```python
from build123d import *

# Parameters (mm, degrees)
ESQUISSE1_W        = 90
ESQUISSE1_H        = 250
BOSS_EXTRU_1_DEPTH = 5
ESQUISSE2_W        = 90
ESQUISSE2_H        = 250
ESQUISSE2_W_2      = 80
ESQUISSE2_H_2      = 240
BOSS_EXTRU_2_DEPTH = 75
BOSS_EXTRU_3_DEPTH = 5


with BuildPart() as part:
    # Esquisse1 → Boss.-Extru.1 (new body)
    with BuildSketch(Plane.XY):
        with Locations((-45, 125)):
            Rectangle(ESQUISSE1_W, ESQUISSE1_H)
    extrude(amount=BOSS_EXTRU_1_DEPTH)

    # Esquisse2 → Boss.-Extru.2 (add)
    with BuildSketch(Plane(origin=(0, 0, 0), x_dir=(-1, 0, 0), z_dir=(0, 0, -1))):
        with Locations((45, 125)):
            Rectangle(ESQUISSE2_W, ESQUISSE2_H)
        with Locations((45, 125)):
            Rectangle(ESQUISSE2_W_2, ESQUISSE2_H_2, mode=Mode.SUBTRACT)
    extrude(amount=BOSS_EXTRU_2_DEPTH)

    # Esquisse3 → Boss.-Extru.3 (add)
    with BuildSketch(Plane(origin=(0, 0, -75), x_dir=(-1, 0, 0), z_dir=(0, 0, -1))):
        Polygon((6.025463364, 250), (-96.347652867, 250), (-96.347652867, 0), (-31.347652867, 0), (45, 0), (45, 5), (5, 5), (5, 245), (45, 245), (45, 250), align=None)
    boss_extru_3 = extrude(amount=BOSS_EXTRU_3_DEPTH)

    # Symétrie1: Boss.-Extru.3 across plane
    add(boss_extru_3.mirror(Plane(origin=(-45, 245, -80), x_dir=(0, 0, 1), z_dir=(1, 0, 0))))


solid = part.part
```
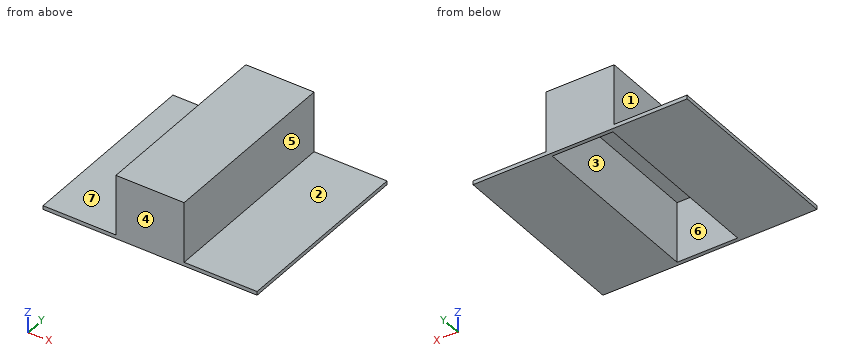
Source: CAD feature listing. Evaluate the final solid. Frame: model axes, mm. Face numbers are marked on the shaded views. A direction names the side the tool comes from. Give positions to 0.01 mm unless a question says otherwise; leave off trailing zeros. Order: outer loops, then holes, each group sorted by start corner. A loop starts at its lowest first (then second) coordinate and runs counter-clockwise, first axis right, second up. Notation, with made-up numbers: (50.5, -29.5) -> (105.5, -29.5) arc R12 ccw to (105.5, -7.5) -> close; hole circle Ø7 at (85, 76). An arc over 180 degrees is marked (long way). Use a Markdown table: item, result.
Q1. Section B-B (y = 50). Return the cut outline in (x, z).
A:
| item | result |
|---|---|
| outline | (-186.35, -80) -> (-85, -80) -> (-85, 0) -> (-5, 0) -> (-5, -80) -> (96.35, -80) -> (96.35, -75) -> (0, -75) -> (0, 5) -> (-90, 5) -> (-90, -75) -> (-186.35, -75) -> close |
Q2. Material intervals for line 1 (X direction, y = 39, z = -30.5); line 2 (Y direction, x = -8, z = -16.5); line 3 (Z direction, x = -44, y = 193.5), sorted ascending. Write a range as [from, to].
A:
| item | result |
|---|---|
| line 1 | [-90, -85], [-5, 0] |
| line 2 | [0, 5], [245, 250] |
| line 3 | [0, 5] |
Q3. Section D-D (x = -143). Return the cut outline in (y, z), and give its area (3 significant figures).
A:
| item | result |
|---|---|
| outline | (0, -80) -> (250, -80) -> (250, -75) -> (0, -75) -> close |
| area | 1,250 mm^2 |
Q4. Access query for the marked faces 4, 5, 6 and 7. Directions: +Z, -Z, +X, -X, +Y, -Y. A direction counts if a zero-diameter tool reaches every point of the face in a straight line with its end or side. Return the directions, or none.
A:
| item | result |
|---|---|
| face 4 | +Z, -Z, +X, -X, -Y |
| face 5 | +Z, +X, +Y, -Y |
| face 6 | -Z |
| face 7 | +Z, -X, +Y, -Y |
Q5. Section A-A (z = -24). Return the cut outline in (x, y), and give its area (3 significant figures).
A:
| item | result |
|---|---|
| outline | (-90, 0) -> (0, 0) -> (0, 250) -> (-90, 250) -> close; hole (-85, 5) -> (-5, 5) -> (-5, 245) -> (-85, 245) -> close |
| area | 3,300 mm^2 |
Q6. Pull-direction query (X, two-part tool) for the marked faces 1, 2 and 3; classes: +X half, -X half, draft (parallel to the pull), parting line (faces both ways), or undercut.
A:
| item | result |
|---|---|
| face 1 | -X half |
| face 2 | draft |
| face 3 | undercut |
Q7. Section C-C (x = -26). Return the cut outline in (y, z), and give its area (3 significant figures).
A:
| item | result |
|---|---|
| outline | (0, -80) -> (5, -80) -> (5, 0) -> (245, 0) -> (245, -80) -> (250, -80) -> (250, 5) -> (0, 5) -> close |
| area | 2,050 mm^2 |
Q8. First-contact query: P1, Ø5, axis at y = 148.5, z = -65.5, coming from the -X side; P2, Ø4, axis at y = 86, z = -60.5, coming from the +X side; P3, Ø4, axis at x = -38.5, y = 45, coming from the -Z side. Flat tips, straight axial feed; report the tip coordinate or a pass-through.
A:
| item | result |
|---|---|
| P1 | x = -90 |
| P2 | x = 0 |
| P3 | z = 0 |
